Verification items for this drawing (mm, ordinates from the low corner). A direction names the side the tool comes from. Round coordinates to 2 decimals unless told otherwise and drop trailing zeros. Loops run counter-clockwise (first coordinate to the right, second up) from the corner with the lowest first, then second, coordinate; pieces in that order, holes last. Notation, with made-up numbers: M -35,52.5 L 14,52.5 A17 ccw 14,56.5 Z; hole C -33.5,-26 d11. An arc over 180 degrees is marked long. Write item = value, one per line. Start each with the question number.
(1) Mould release check, pull along X, two halves, no side actions. Record for the marked faces 1, 2 and 3: pulls with the +X half, pulls with the -X half, needs draft (parallel to the pull), parting line crosses it, or undercut.
(2) Set-up check for the marked faces 4, 5 and 6: record each of +Z, -Z, +X, -X, +Y, -Y from which the full face is reachable in a straight line by a thin tool's end or side.
(3) Cross-section at C-C on z = 3.25. Record the boundary of the cut face in (x, y), plus the area to 3 significant figures.
(4) Cross-section at A-A on y = 11. Record the boundary of the cut face in (x, z).
(5) Go/stop test with flat-tipped pins: P1, Ø1.5, axis at x = 17, z = 2.5, coming from the +Y side; P2, Ø2, axis at x = 18.5, y = 12.5, coming from the +Z side. Record where each tip stops, or that it passes through.
(6) Cross-section at D-D on x = 5.5. Record the boundary of the cut face in (y, z), plus the area to 3 significant figures.
(7) Scan lines: L1, parallel to Y at x = 11, z = 0.3; L2, parallel to Y at x = 11, z = 3.75; L3, parallel to Z at x = 13, y = 4.25. Record each from-to range of solid material in increasing order. Write a range as from..to.
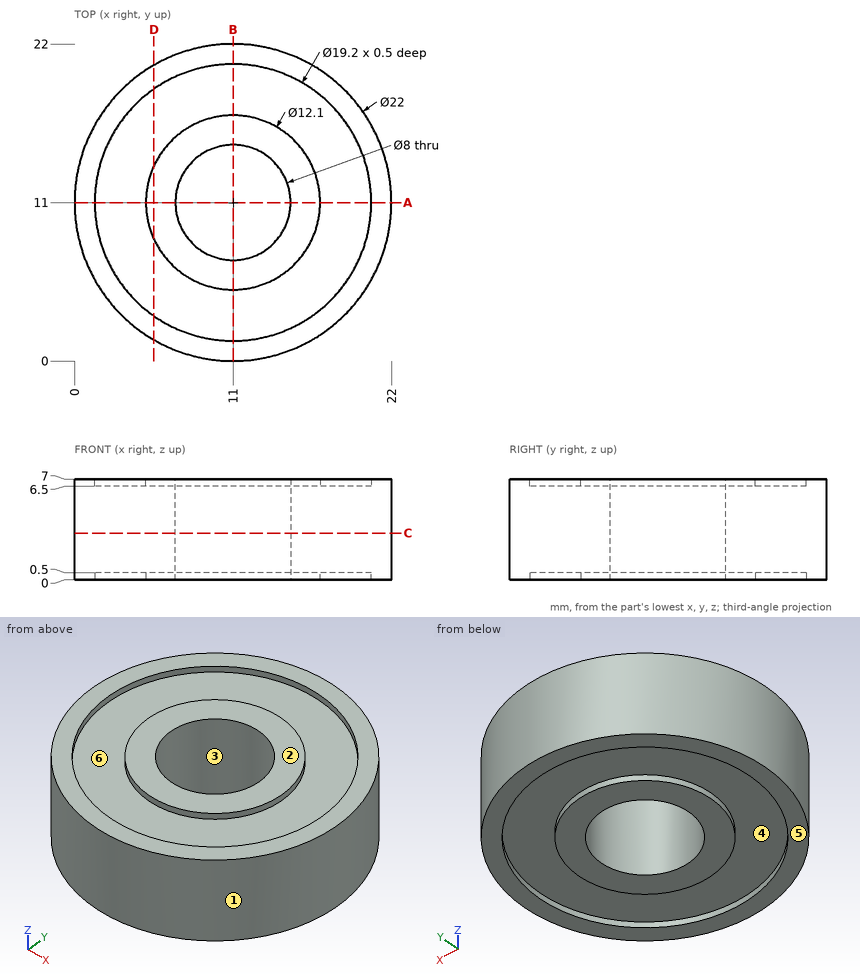
Result:
q1.face_1 = parting line crosses it
q1.face_2 = needs draft
q1.face_3 = undercut
q2.face_4 = -Z
q2.face_5 = -Z, +X, -X, +Y, -Y
q2.face_6 = +Z
q3.outline = C 11,11 d22; hole C 11,11 d8
q3.area = 330 mm^2
q4.outline = M 0,0 L 1.4,0 L 1.4,0.5 L 4.95,0.5 L 4.95,0 L 7,0 L 7,7 L 4.95,7 L 4.95,6.5 L 1.4,6.5 L 1.4,7 L 0,7 Z; M 15,0 L 17.05,0 L 17.05,0.5 L 20.6,0.5 L 20.6,0 L 22,0 L 22,7 L 20.6,7 L 20.6,6.5 L 17.05,6.5 L 17.05,7 L 15,7 Z
q5.P1 = 20.67
q5.P2 = 6.5
q6.outline = M 1.47,0 L 3.13,0 L 3.13,0.5 L 8.48,0.5 L 8.48,0 L 13.52,0 L 13.52,0.5 L 18.87,0.5 L 18.87,0 L 20.53,0 L 20.53,7 L 18.87,7 L 18.87,6.5 L 13.52,6.5 L 13.52,7 L 8.48,7 L 8.48,6.5 L 3.13,6.5 L 3.13,7 L 1.47,7 Z
q6.area = 123 mm^2
q7.L1 = 0..1.4, 4.95..7, 15..17.05, 20.6..22
q7.L2 = 0..7, 15..22
q7.L3 = 0.5..6.5
